from build123d import *

# Parameters (mm, degrees)
F0_R     = 9
F1_DEPTH = 3
F2_SIZE  = 0.5
F3_R     = 4
F4_DEPTH = 4
F5_R     = 2.5
F6_DEPTH = 3
F8_DEPTH = 1.5


with BuildPart() as f1:
    # F0 (on Top) → F1 (new body)
    with BuildSketch(Plane.XY):
        Circle(F0_R)
    extrude(amount=F1_DEPTH)

    # F2
    f2_edges = [f1.edges().sort_by_distance(p)[0] for p in [
        (-9, 0, 3),
    ]]
    chamfer(f2_edges, length=F2_SIZE)

    # F3 (on face) → F4 (join)
    with BuildSketch(Plane.XY.offset(3)):
        Circle(F3_R)
    extrude(amount=F4_DEPTH)

    # F5 (on face) → F6 (join)
    with BuildSketch(Plane.XY.offset(7)):
        Circle(F5_R)
    extrude(amount=F6_DEPTH)

    # F7 (on face) → F8 (cut)
    with BuildSketch(Plane(origin=(0, 0, 0), x_dir=(1, 0, 0), z_dir=(0, 0, -1))):
        Polygon((-0.031379, 5.948377), (-0.235333, 5.919157), (-0.372759, 5.868757), (-0.500818, 5.801363), (-0.64831, 5.683569), (-0.711513, 5.643549), (-0.766303, 5.595223), (-0.884297, 5.389084), (-0.972792, 2.355883), (-1.91674, 3.298237), (-2.464657, 3.842872), (-2.74588, 4.106761), (-3.037677, 4.358384), (-3.197437, 4.424921), (-3.362159, 4.476179), (-3.5244, 4.487041), (-3.686641, 4.476179), (-4.011123, 4.358384), (-4.276609, 4.122796), (-4.349034, 4.030994), (-4.401972, 3.928468), (-4.483097, 3.710516), (-4.483097, 3.357134), (-4.394602, 3.092097), (-4.24711, 2.885957), (-3.303163, 1.914155), (-2.359215, 0.971802), (-5.220556, 0.942353), (-5.397547, 0.883456), (-5.427045, 0.854008), (-5.556038, 0.793243), (-5.614945, 0.756011), (-5.663032, 0.706765), (-5.840022, 0.471176), (-5.958016, 0.117794), (-5.958016, -0.058897), (-5.940408, -0.209293), (-5.899019, -0.353383), (-5.843566, -0.461413), (-5.781025, -0.559523), (-5.655249, -0.699811), (-5.51554, -0.82456), (-5.220556, -0.942354), (-5.075648, -0.968558), (-4.928112, -0.97628), (-4.630589, -0.971802), (-4.188114, -0.971802), (-2.359215, -0.971802), (-2.368134, -1.005446), (-2.388713, -1.030699), (-3.332661, -1.973053), (-4.276609, -2.915406), (-4.34313, -2.999393), (-4.394602, -3.092097), (-4.419005, -3.155066), (-4.453599, -3.209892), (-4.476923, -3.415726), (-4.483097, -3.622171), (-4.464349, -3.757662), (-4.424101, -3.887208), (-4.374765, -3.997645), (-4.306107, -4.093348), (-4.188114, -4.240591), (-4.103985, -4.307), (-4.011123, -4.358385), (-3.71614, -4.476179), (-3.391658, -4.476179), (-3.067176, -4.387833), (-2.890186, -4.240591), (-1.946238, -3.298237), (-1.00229, -2.355884), (-0.884297, -5.418533), (-0.8253, -5.506878), (-0.699524, -5.647167), (-0.559815, -5.771915), (-0.503448, -5.807594), (-0.441821, -5.830812), (-0.341941, -5.885287), (-0.235333, -5.919158), (0.089149, -5.948606), (0.384133, -5.889709), (0.708615, -5.654121), (0.754319, -5.61094), (0.790702, -5.558969), (0.856107, -5.447981), (0.9741, -5.094599), (0.9741, -4.417282), (0.9741, -2.591472), (0.971489, -2.477691), (0.979459, -2.426523), (1.003599, -2.385332), (1.947546, -3.327686), (2.891494, -4.270039), (3.122896, -4.385014), (3.363468, -4.476179), (3.68795, -4.476179), (3.805943, -4.446731), (3.94337, -4.39633), (4.071429, -4.328936), (4.218921, -4.211142), (4.425409, -3.916657), (4.513904, -3.474929), (4.444862, -3.229831), (4.398065, -3.113042), (4.336914, -3.003752), (4.300041, -2.947904), (4.277917, -2.885958), (3.33397, -1.943604), (2.390022, -1.001251), (2.41952, -0.971802), (2.861996, -0.971802), (4.690894, -0.971802), (4.972609, -0.968567), (5.251363, -0.942354), (5.280862, -0.912905), (5.546347, -0.82456), (5.723337, -0.61842), (5.839817, -0.478169), (5.883167, -0.404005), (5.900327, -0.323934), (5.934856, -0.237188), (5.954737, -0.147151), (5.958016, 0.039233), (5.925076, 0.228087), (5.870829, 0.412279), (5.7562, 0.594983), (5.685681, 0.672036), (5.605344, 0.736213), (5.428354, 0.883456), (5.192367, 0.942353), (4.838344, 0.987761), (4.482387, 1.011028), (3.766457, 1.011578), (3.048146, 0.984877), (2.331025, 0.971802), (3.274973, 1.914155), (4.218921, 2.856509), (4.337268, 2.979647), (4.379451, 3.047229), (4.395911, 3.121546), (4.454907, 3.209891), (4.513904, 3.504377), (4.444233, 3.827854), (4.386266, 3.98061), (4.307416, 4.122796), (4.04193, 4.358384), (3.717448, 4.476179), (3.555567, 4.481563), (3.392966, 4.476179), (3.215976, 4.44673), (3.186478, 4.417282), (3.038986, 4.358384), (2.944209, 4.294123), (2.861996, 4.211142), (1.918048, 3.268788), (0.9741, 2.326435), (0.9741, 3.092097), (0.9741, 4.947355), (0.94889, 5.186814), (0.885605, 5.418532), (0.649618, 5.713018), (0.576669, 5.769819), (0.540299, 5.792295), (0.502126, 5.801363), (0.468426, 5.810267), (0.44313, 5.830812), (0.313926, 5.898818), (0.177644, 5.948606), align=None)
    extrude(amount=-F8_DEPTH, mode=Mode.SUBTRACT)


solid = f1.part
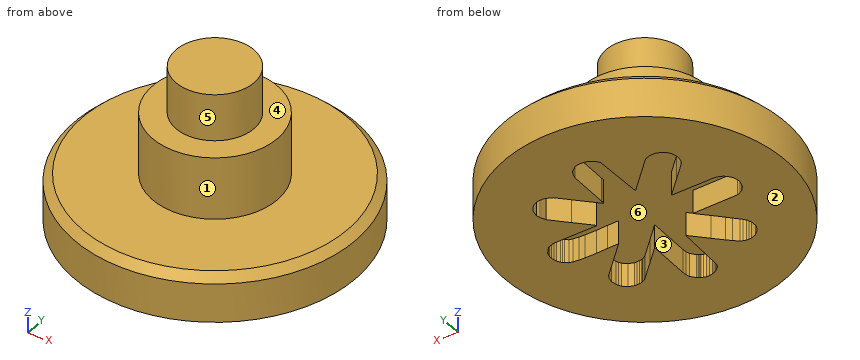
Could you check a few things on this model? Use its own coordinates, in mm. Face numbers are marked on the shaded views. A direction names the side the tool comes from. Round coordinates to 2 decimals unless told otherwise and drop trailing zeros. Order: outer loops, then holes, each group sorted by start corner. A loop starts at its lowest first (then second) coordinate and runs counter-clockwise, first axis right, second up.
Q1. Which directions (+Z, -Z, +X, -X, +Y, -Y) give clear straight access to the entire face, cutting with the end or side of a thin tool? Please do the marked faces 1, 2 and 3.
Geometry says:
face 1: +Z
face 2: -Z, +X, -X, +Y, -Y
face 3: -Z
Q2. Imagine slicing it at B-B, the plane z = 5.25. List the corners of the cut face in (x, y) for me, then the cut area to 3 significant figures.
Geometry says:
outline: circle Ø8 at (0, 0)
area: 50.3 mm2
Q3. Thinking about a two-plate mould opening in Y: for the marked faces 4, 5 and 6, which applies, released by +Y, released by -Y, zero draft, split by the parting line, or undercut?
Geometry says:
face 4: zero draft
face 5: split by the parting line
face 6: undercut
Q4. Imagine slicing it at A-A, the plane z = 2. List the corners of the cut face in (x, y) for me, then the cut area to 3 significant figures.
Geometry says:
outline: circle Ø18 at (0, 0)
area: 254 mm2
Q5. Please list where these lines run through material, in increasing order: probe 1 along Y at (x, z) = (-3.5, 1); probe 2 along Z at (x, y) = (2, -5); probe 3 along Z at (x, y) = (-1.5, 2.5).
Geometry says:
probe 1: y = -8.29 to -4.49, -2.12 to -0.96, 0.97 to 2.14, 4.48 to 8.29
probe 2: z = 0 to 3
probe 3: z = 1.5 to 7
Q6. I'm going to push flat-ended pins straight in: P1, Ø3, axis at x = 0.5, z = 6.5, coming from the +Y side; P2, Ø3, axis at x = -2, z = 8, coming from the -Y side; P3, Ø1, axis at y = -0.5, z = 5, coming from the -X side. Where does each tip first touch, or does it pass through?
Geometry says:
P1: stops at y = 4
P2: stops at y = -3.9
P3: stops at x = -4
